from build123d import *

# Parameters (mm, degrees)
SKETCH1_R           = 1.6
BOSS_EXTRUDE1_DEPTH = 2.8
CUT_EXTRUDE2_START  = 2.8
SKETCH1_6_R         = 2.1
CUT_EXTRUDE2_DEPTH  = 1.8
CHAMFER1_SIZE       = 1.5
CHAMFER1_SIZE_2     = 2
FILLET1_START       = -33.224011807
FILLET1_DEPTH       = 66.448023614
FILLET1_START_2     = -38.224011807
FILLET1_2_DEPTH     = 76.3236742


with BuildPart() as part:
    # Sketch1 → Boss-Extrude1 (new body)
    with BuildSketch(Plane(origin=(0, 0, 0), x_dir=(0, 1, 0), z_dir=(0, 0, 1))):
        with BuildLine():
            Line((31.25, 38.25), (-31.25, 38.25))
            ThreePointArc((-31.25, 38.25), (-32.664213562, 37.664213562), (-33.25, 36.25))
            Line((-33.25, 36.25), (-33.25, -36.25))
            ThreePointArc((-33.25, -36.25), (-32.664213562, -37.664213562), (-31.25, -38.25))
            Line((-31.25, -38.25), (31.25, -38.25))
            ThreePointArc((31.25, -38.25), (32.664213562, -37.664213562), (33.25, -36.25))
            Line((33.25, -36.25), (33.25, 36.25))
            ThreePointArc((33.25, 36.25), (32.664213562, 37.664213562), (31.25, 38.25))
        make_face()
        with Locations(Location((-30.75, -35.75, 0), (0, 0, 270))):
            Circle(SKETCH1_R, mode=Mode.SUBTRACT)
        with Locations(Location((30.75, -35.75, 0), (0, 0, 270))):
            Circle(SKETCH1_R, mode=Mode.SUBTRACT)
        with BuildLine():
            ThreePointArc((-28.5, 10), (-27.914213562, 11.414213562), (-26.5, 12))
            Line((-26.5, 12), (-13.5, 12))
            ThreePointArc((-13.5, 12), (-12.085786438, 11.414213562), (-11.5, 10))
            Line((-11.5, 10), (-11.5, -10))
            ThreePointArc((-11.5, -10), (-12.085786438, -11.414213562), (-13.5, -12))
            Line((-13.5, -12), (-26.5, -12))
            ThreePointArc((-26.5, -12), (-27.914213562, -11.414213562), (-28.5, -10))
            Line((-28.5, -10), (-28.5, 10))
        make_face(mode=Mode.SUBTRACT)
        with Locations(Location((-30.75, 35.75, 0), (0, 0, 270))):
            Circle(SKETCH1_R, mode=Mode.SUBTRACT)
        with BuildLine():
            Line((-10.5, -27), (-10.5, 27))
            ThreePointArc((-10.5, 27), (-9.914213562, 28.414213562), (-8.5, 29))
            Line((-8.5, 29), (8.5, 29))
            ThreePointArc((8.5, 29), (9.914213562, 28.414213562), (10.5, 27))
            Line((10.5, 27), (10.5, -27))
            ThreePointArc((10.5, -27), (9.914213562, -28.414213562), (8.5, -29))
            Line((8.5, -29), (-8.5, -29))
            ThreePointArc((-8.5, -29), (-9.914213562, -28.414213562), (-10.5, -27))
        make_face(mode=Mode.SUBTRACT)
        with Locations(Location((30.75, 35.75, 0), (0, 0, 270))):
            Circle(SKETCH1_R, mode=Mode.SUBTRACT)
    extrude(amount=BOSS_EXTRUDE1_DEPTH)

    # Sketch1<6> → Cut-Extrude2 (cut)
    with BuildSketch(Plane(origin=(0, 0, 0), x_dir=(0, 1, 0), z_dir=(0, 0, 1)).offset(CUT_EXTRUDE2_START)):
        with Locations(Location((-23, 33, 0), (0, 0, 270))):
            Circle(SKETCH1_6_R)
        with Locations(Location((23, 33, 0), (0, 0, 270))):
            Circle(SKETCH1_6_R)
        with Locations(Location((23, -33, 0), (0, 0, 270))):
            Circle(SKETCH1_6_R)
        with Locations(Location((-23, -33, 0), (0, 0, 270))):
            Circle(SKETCH1_6_R)
    extrude(amount=-CUT_EXTRUDE2_DEPTH, mode=Mode.SUBTRACT)

    # Cut-Extrude1 cone 1 section (through the dimple's axis) → Cut-Extrude1 (revolve, cut)
    with BuildSketch(Plane(origin=(33, -23, 1), x_dir=(0, -1, 0), z_dir=(1, 0, 0))):
        Polygon((0, 0), (1.1, 0), (0, 12.573057533), align=None)
    revolve(axis=Axis((33, -23, 1), (0, 0, -1)), mode=Mode.SUBTRACT)

    # Cut-Extrude1 cone 2 section (through the dimple's axis) → Cut-Extrude1 cone 2 (revolve, cut)
    with BuildSketch(Plane(origin=(-33, -23, 1), x_dir=(0, -1, 0), z_dir=(1, 0, 0))):
        Polygon((0, 0), (1.1, 0), (0, 12.573057533), align=None)
    revolve(axis=Axis((-33, -23, 1), (0, 0, -1)), mode=Mode.SUBTRACT)

    # Cut-Extrude1 cone 3 section (through the dimple's axis) → Cut-Extrude1 cone 3 (revolve, cut)
    with BuildSketch(Plane(origin=(-33, 23, 1), x_dir=(0, -1, 0), z_dir=(1, 0, 0))):
        Polygon((0, 0), (1.1, 0), (0, 12.573057533), align=None)
    revolve(axis=Axis((-33, 23, 1), (0, 0, -1)), mode=Mode.SUBTRACT)

    # Cut-Extrude1 cone 4 section (through the dimple's axis) → Cut-Extrude1 cone 4 (revolve, cut)
    with BuildSketch(Plane(origin=(33, 23, 1), x_dir=(0, -1, 0), z_dir=(1, 0, 0))):
        Polygon((0, 0), (1.1, 0), (0, 12.573057533), align=None)
    revolve(axis=Axis((33, 23, 1), (0, 0, -1)), mode=Mode.SUBTRACT)

    # Chamfer1
    # the kernel refuses this chamfer: 2, 1.5 mm, written as the material it takes off along each edge
    with BuildSketch(Plane(origin=(-35.75, -30.75, 2.8), x_dir=(1, 0, 0), z_dir=(0, -1, 0))) as chamfer1_piece_1:
        Polygon((1.6 + CHAMFER1_SIZE, 0), (1.6, -CHAMFER1_SIZE_2), (1.6, 0), align=None)
    revolve(axis=Axis((-35.75, -30.75, 2.8), (0, 0, 1)), mode=Mode.SUBTRACT)
    with BuildSketch(Plane(origin=(35.75, -30.75, 2.8), x_dir=(1, 0, 0), z_dir=(0, -1, 0))) as chamfer1_piece_2:
        Polygon((1.6 + CHAMFER1_SIZE, 0), (1.6, -CHAMFER1_SIZE_2), (1.6, 0), align=None)
    revolve(axis=Axis((35.75, -30.75, 2.8), (0, 0, 1)), mode=Mode.SUBTRACT)
    with BuildSketch(Plane(origin=(35.75, 30.75, 2.8), x_dir=(1, 0, 0), z_dir=(0, -1, 0))) as chamfer1_piece_3:
        Polygon((1.6 + CHAMFER1_SIZE, 0), (1.6, -CHAMFER1_SIZE_2), (1.6, 0), align=None)
    revolve(axis=Axis((35.75, 30.75, 2.8), (0, 0, 1)), mode=Mode.SUBTRACT)
    with BuildSketch(Plane(origin=(-35.75, 30.75, 2.8), x_dir=(1, 0, 0), z_dir=(0, -1, 0))) as chamfer1_piece_4:
        Polygon((1.6 + CHAMFER1_SIZE, 0), (1.6, -CHAMFER1_SIZE_2), (1.6, 0), align=None)
    revolve(axis=Axis((-35.75, 30.75, 2.8), (0, 0, 1)), mode=Mode.SUBTRACT)

    # Fillet1: read off the stored shape, not the designer's step
    # Fillet1 outline → Fillet1 (cut)
    with BuildSketch(Plane(origin=(0, 0, 0), x_dir=(1, 0, 0), z_dir=(0, 1, 0)).offset(FILLET1_START)):
        with BuildLine():
            ThreePointArc((38.25, -1.8), (37.957106781, -2.507106781), (37.25, -2.8))
            Line((37.25, -2.8), (38.25, -2.8))
            Line((38.25, -2.8), (38.25, -1.8))
        make_face()
        with BuildLine():
            ThreePointArc((-37.25, -2.8), (-37.957106781, -2.507106781), (-38.25, -1.8))
            Line((-38.25, -1.8), (-38.25, -2.8))
            Line((-38.25, -2.8), (-37.25, -2.8))
        make_face()
    extrude(amount=FILLET1_DEPTH, mode=Mode.SUBTRACT)

    # Fillet1 2 outline → Fillet1 2 (cut)
    with BuildSketch(Plane.YZ.offset(FILLET1_START_2)):
        with BuildLine():
            Line((-33.25, 2.8), (-33.25, 1.8))
            ThreePointArc((-33.25, 1.8), (-32.957106781, 2.507106781), (-32.25, 2.8))
            Line((-32.25, 2.8), (-33.25, 2.8))
        make_face()
        with BuildLine():
            Line((33.25, 2.8), (32.25, 2.8))
            ThreePointArc((32.25, 2.8), (32.957106781, 2.507106781), (33.25, 1.8))
            Line((33.25, 1.8), (33.25, 2.8))
        make_face()
    extrude(amount=FILLET1_2_DEPTH, mode=Mode.SUBTRACT)


solid = part.part
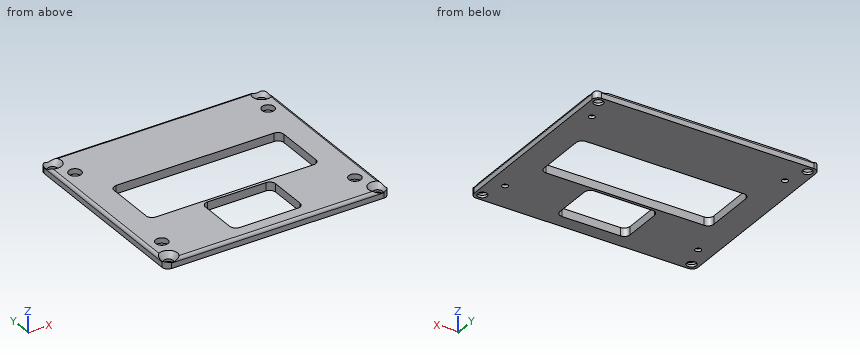
Can you work these out from the model? Positions are in its coordinate system, mm. Give positions to 0.01 mm unless a question says otherwise; leave off trailing zeros. Loops run counter-clockwise (first coordinate to the right, second up) from the corner with the lowest first, then second, coordinate; pieces in that order, holes last. Notation, with made-up numbers: (33.25, 81.25) - (51.25, 81.25) arc R25 cw to (51.25, 95.25) - close; hole circle Ø4 at (32.25, 89). An arc over 180 degrees is marked (long way). One line per item, written item: value.
(1) If we section it at A-A, the plane x = 24: List the corners of the cut face in (y, z) for me.
Verdict:
outline: (-33.25, 0) - (-10.5, 0) - (-10.5, 2.8) - (-32.25, 2.8) arc R1 ccw to (-33.25, 1.8) - close; (10.5, 0) - (33.25, 0) - (33.25, 1.8) arc R1 ccw to (32.25, 2.8) - (10.5, 2.8) - close
(2) If we section it at B-B, the plane y = 4: List the corners of the cut face in (x, z) for me, plus the area to 3 significant figures.
Verdict:
outline: (-38.25, 0) - (-29, 0) - (-29, 2.8) - (-37.25, 2.8) arc R1 ccw to (-38.25, 1.8) - close; (29, 0) - (38.25, 0) - (38.25, 1.8) arc R1 ccw to (37.25, 2.8) - (29, 2.8) - close
area: 51.4 mm^2
(3) If we section it at C-C, the plane y = -23: List the corners of the cut face in (x, z) for me, plus the area to 3 significant figures.
Verdict:
outline: (-38.25, 0) - (-34.01, 0) - (-34.1, 1) - (-35.1, 1) - (-35.1, 2.8) - (-37.25, 2.8) arc R1 ccw to (-38.25, 1.8) - close; (-31.99, 0) - (-12, 0) - (-12, 2.8) - (-30.9, 2.8) - (-30.9, 1) - (-31.9, 1) - close; (12, 0) - (31.99, 0) - (31.9, 1) - (30.9, 1) - (30.9, 2.8) - (12, 2.8) - close; (34.01, 0) - (38.25, 0) - (38.25, 1.8) arc R1 ccw to (37.25, 2.8) - (35.1, 2.8) - (35.1, 1) - (34.1, 1) - close
area: 127 mm^2
(4) I need wall thicknesses on line 1 along Y through (x, z) = (35.75, 0.25); line 2 along Y through (x, z) = (33, 1.65); line 3 along X through (y, z) = (-4.5, 0.4). Which ranges of each line are inside material? Lowest first, please.
Verdict:
line 1: -33.25 to -32.35, -29.15 to 29.15, 32.35 to 33.25
line 2: -33.25 to -25.1, -20.9 to 20.9, 25.1 to 33.25
line 3: -38.25 to -29, 29 to 38.25
(5) I'm going to push flat-ended pins straight in: pin 1 (1.3 mm diameter, centred on x = -34, y = -24, fed in from +Z); pin 2 (3 mm diameter, centred on x = 21.5, y = 26, fed in from -Z); pin 3 (1.9 mm diameter, centred on x = -35.75, y = 30.75, fed in from +Z); pin 4 (5 mm diameter, centred on x = 35.75, y = -30.75, fed in from +Z). Where does each tip first touch, or does it pass through?
Verdict:
pin 1: z = 1
pin 2: z = 0
pin 3: through
pin 4: z = 2
